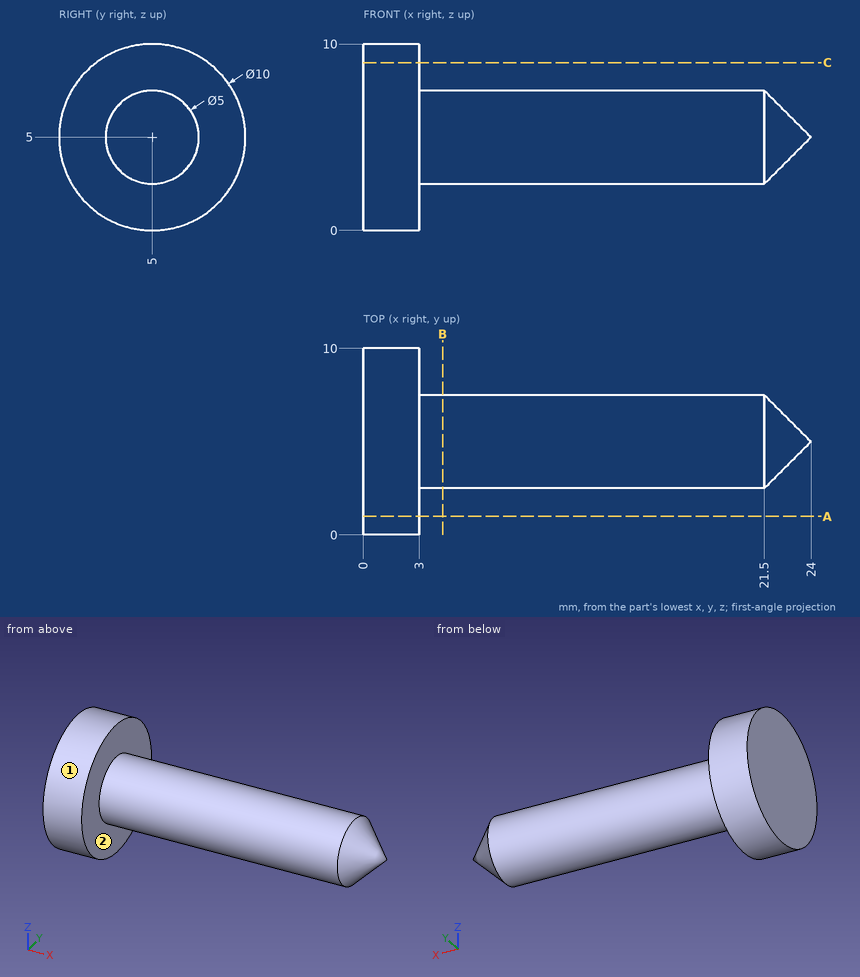
Answer from the drawing. Dimensions are ordinates in mm from the lowest x, y and z of the part. A direction names the side the tool comes from. Round coordinates to 2 decimals unless told otherwise and drop trailing zeros. Order: outer loops, then holes, each group sorted by start corner. A loop starts at its lowest first (then second) coordinate and runs counter-clockwise, first axis right, second up.
1) For the marked faces 1 and 2, determine the directions among +Z, -Z, +X, -X, +Y, -Y from which every point of the face is accessible in a straight line to the end or side of a thin tool.
2) The part is cut by section A-A on y = 1. Write down the section's boundary in (x, z), plus the area to 3 significant figures.
3) The part is cut by section B-B on x = 4.25. Write down the section's boundary in (y, z), plus the area to 3 significant figures.
4) Straight lines are drawn through the part: L1, parallel to X at y = 9.25, z = 7.5; L2, parallel to X at y = 5, z = 3.25; L3, parallel to Z at x = 11.25, y = 3.5. For each, find the intervals that lie inside material, in ascending order.
5) Flat-ended cylindrical pins translate along their axes: pin 1 (3 mm diameter, centred on y = 6, z = 7, fed in from +X); pin 2 (5 mm diameter, centred on y = 6.5, z = 8.5, fed in from +X); pin 3 (1 mm diameter, centred on y = 4.5, z = 3, fed in from +X). Find the tip coordinate at first contact, or state that the pin passes through.
Resolved:
1. face 1: +X, -X
1. face 2: +X
2. outline: (0, 2) - (3, 2) - (3, 8) - (0, 8) - close
2. area: 18.0 mm2
3. outline: circle Ø5 at (5, 5)
3. area: 19.6 mm2
4. L1: x = 0 to 3
4. L2: x = 0 to 22.25
4. L3: z = 3 to 7
5. pin 1: stops at x = 23.26
5. pin 2: stops at x = 22.69
5. pin 3: stops at x = 22.44
